Build history of the part. All positions in model axes, mm. Face numbers are marked on the shaded views. A direction names the side the tool comes from. Give positions to 0.01 mm unless a question says otherwise; leave off trailing zeros. Order: outer loops, then holes, each group sorted by start corner. A loop starts at its lowest first (then second) coordinate and runs counter-clockwise, first axis right, second up. Notation, with made-up numbers: (20.5, 64.5) - (70.5, 64.5) arc R7 cw to (70.5, 68.5) - close; hole circle Ø1 at (84, -39). An arc over 180 degrees is marked (long way). Use a Markdown table: item, result.
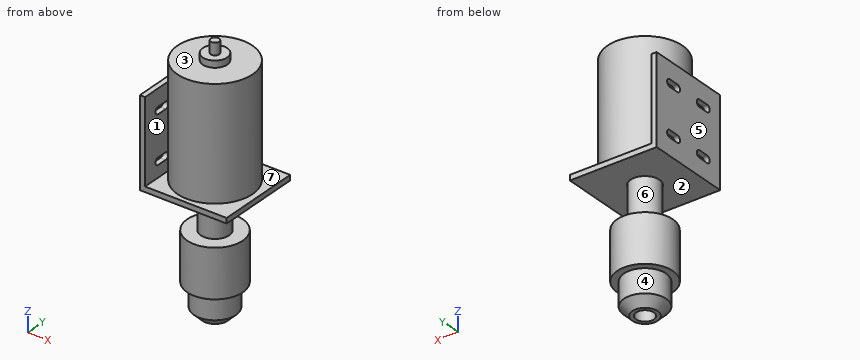
from build123d import *

# Parameters (mm, degrees)
SKETCH1_R           = 22.25
BOSS_EXTRUDE1_DEPTH = 66
SKETCH2_R           = 7.25
BOSS_EXTRUDE2_DEPTH = 4
SKETCH3_R           = 2.5
BOSS_EXTRUDE3_DEPTH = 7
SKETCH4_W           = 51.5
SKETCH4_H           = 50
SKETCH4_R           = 8.6
BOSS_EXTRUDE4_DEPTH = 3.1
SKETCH5_R           = 8.4
BOSS_EXTRUDE5_DEPTH = 27.7
SKETCH6_R           = 16.5
BOSS_EXTRUDE6_DEPTH = 28.5
SKETCH7_R           = 12.5
BOSS_EXTRUDE7_DEPTH = 18.9
SKETCH8_R           = 5.3
CUT_EXTRUDE1_DEPTH  = 26.4
CHAMFER1_SIZE       = 5
SKETCH9_W           = 3.1
SKETCH9_H           = 50
BOSS_EXTRUDE8_DEPTH = 49.3
CUT_EXTRUDE2_REACH  = 53.5


with BuildPart() as part:
    # Sketch1 → Boss-Extrude1 (new body)
    with BuildSketch(Plane.XY):
        Circle(SKETCH1_R)
    extrude(amount=BOSS_EXTRUDE1_DEPTH)

    # Sketch2 → Boss-Extrude2 (add)
    with BuildSketch(Plane.XY.offset(66)):
        Circle(SKETCH2_R)
    extrude(amount=BOSS_EXTRUDE2_DEPTH)

    # Sketch3 → Boss-Extrude3 (add)
    with BuildSketch(Plane.XY.offset(70)):
        Circle(SKETCH3_R)
    extrude(amount=BOSS_EXTRUDE3_DEPTH)

    # Sketch4 → Boss-Extrude4 (add)
    with BuildSketch(Plane(origin=(0, 0, 0), x_dir=(-1, 0, 0), z_dir=(0, 0, -1))):
        Rectangle(SKETCH4_W, SKETCH4_H)
        Circle(SKETCH4_R, mode=Mode.SUBTRACT)
    extrude(amount=BOSS_EXTRUDE4_DEPTH)

    # Sketch5 → Boss-Extrude5 (add)
    with BuildSketch(Plane(origin=(0, 0, 0), x_dir=(-1, 0, 0), z_dir=(0, 0, -1))):
        Circle(SKETCH5_R)
    extrude(amount=BOSS_EXTRUDE5_DEPTH)

    # Sketch6 → Boss-Extrude6 (add)
    with BuildSketch(Plane(origin=(0, 0, -27.7), x_dir=(-1, 0, 0), z_dir=(0, 0, -1))):
        Circle(SKETCH6_R)
    extrude(amount=BOSS_EXTRUDE6_DEPTH)

    # Sketch7 → Boss-Extrude7 (add)
    with BuildSketch(Plane(origin=(0, 0, -56.2), x_dir=(-1, 0, 0), z_dir=(0, 0, -1))):
        Circle(SKETCH7_R)
    extrude(amount=BOSS_EXTRUDE7_DEPTH)

    # Sketch8 → Cut-Extrude1 (cut)
    with BuildSketch(Plane(origin=(0, 0, -75.1), x_dir=(-1, 0, 0), z_dir=(0, 0, -1))):
        Circle(SKETCH8_R)
    extrude(amount=-CUT_EXTRUDE1_DEPTH, mode=Mode.SUBTRACT)

    # Chamfer1
    chamfer1_edges = [part.edges().sort_by_distance(p)[0] for p in [
        (12.5, 0, -75.1),
    ]]
    chamfer(chamfer1_edges, length=CHAMFER1_SIZE)

    # Sketch9 → Boss-Extrude8 (add)
    with BuildSketch(Plane.XY):
        with Locations((-24.2, 0)):
            Rectangle(SKETCH9_W, SKETCH9_H)
    extrude(amount=BOSS_EXTRUDE8_DEPTH)

    # Sketch10 → Cut-Extrude2 (cut, up to next)
    with BuildSketch(Plane.ZY.offset(25.75), mode=Mode.PRIVATE) as cut_extrude2_sk1:
        with BuildLine():
            Line((39.2, 14.7), (39.2, 8.7))
            ThreePointArc((39.2, 8.7), (37.1, 6.6), (35, 8.7))
            Line((35, 8.7), (35, 14.7))
            ThreePointArc((35, 14.7), (37.1, 16.8), (39.2, 14.7))
        make_face()
    cut_extrude2_tool1 = extrude(cut_extrude2_sk1.sketch, amount=-CUT_EXTRUDE2_REACH, mode=Mode.PRIVATE) & part.part
    add(cut_extrude2_tool1.solids().sort_by_distance((-25.75, 11.7, 37.1))[0], mode=Mode.SUBTRACT)
    # Sketch10 → Cut-Extrude2 (cut, up to next)
    with BuildSketch(Plane.ZY.offset(25.75), mode=Mode.PRIVATE) as cut_extrude2_sk2:
        with BuildLine():
            Line((39.2, -14.7), (39.2, -8.7))
            ThreePointArc((39.2, -8.7), (37.1, -6.6), (35, -8.7))
            Line((35, -8.7), (35, -14.7))
            ThreePointArc((35, -14.7), (37.1, -16.8), (39.2, -14.7))
        make_face()
    cut_extrude2_tool2 = extrude(cut_extrude2_sk2.sketch, amount=-CUT_EXTRUDE2_REACH, mode=Mode.PRIVATE) & part.part
    add(cut_extrude2_tool2.solids().sort_by_distance((-25.75, -11.7, 37.1))[0], mode=Mode.SUBTRACT)
    # Sketch10 → Cut-Extrude2 (cut, up to next)
    with BuildSketch(Plane.ZY.offset(25.75), mode=Mode.PRIVATE) as cut_extrude2_sk3:
        with BuildLine():
            Line((7, -14.7), (7, -8.7))
            ThreePointArc((7, -8.7), (9.1, -6.6), (11.2, -8.7))
            Line((11.2, -8.7), (11.2, -14.7))
            ThreePointArc((11.2, -14.7), (9.1, -16.8), (7, -14.7))
        make_face()
    cut_extrude2_tool3 = extrude(cut_extrude2_sk3.sketch, amount=-CUT_EXTRUDE2_REACH, mode=Mode.PRIVATE) & part.part
    add(cut_extrude2_tool3.solids().sort_by_distance((-25.75, -11.7, 9.1))[0], mode=Mode.SUBTRACT)
    # Sketch10 → Cut-Extrude2 (cut, up to next)
    with BuildSketch(Plane.ZY.offset(25.75), mode=Mode.PRIVATE) as cut_extrude2_sk4:
        with BuildLine():
            Line((7, 14.7), (7, 8.7))
            ThreePointArc((7, 8.7), (9.1, 6.6), (11.2, 8.7))
            Line((11.2, 8.7), (11.2, 14.7))
            ThreePointArc((11.2, 14.7), (9.1, 16.8), (7, 14.7))
        make_face()
    cut_extrude2_tool4 = extrude(cut_extrude2_sk4.sketch, amount=-CUT_EXTRUDE2_REACH, mode=Mode.PRIVATE) & part.part
    add(cut_extrude2_tool4.solids().sort_by_distance((-25.75, 11.7, 9.1))[0], mode=Mode.SUBTRACT)


solid = part.part
1) Slice it at A-A (z = 37.1). Write the cut outline in (x, y).
Computed:
| item | result |
|---|---|
| outline | (-25.75, -25) - (-22.65, -25) - (-22.65, -16.8) - (-25.75, -16.8) - close; (-25.75, -6.6) - (-22.65, -6.6) - (-22.65, 6.6) - (-25.75, 6.6) - close; (-25.75, 16.8) - (-22.65, 16.8) - (-22.65, 25) - (-25.75, 25) - close; circle Ø44.5 at (0, 0) |
2) Wall check: line 1 (Y direction, x = 0, z = -1); line 2 (Z direction, x = -15, y = 4.5); line 3 (Y direction, x = 0, z = -57.25). Give the ranges that are in metal, low to high. Write a range as from..to.
Computed:
| item | result |
|---|---|
| line 1 | y = -25..-8.6, -8.4..8.4, 8.6..25 |
| line 2 | z = -56.2..-27.7, -3.1..66 |
| line 3 | y = -12.5..-5.3, 5.3..12.5 |
3) Pin check, flat tips, straight feed: P1, Ø0.9, axis at x = -25, y = -11.5, coming from the -Z side; P2, Ø5, axis at x = -0.5, y = -3.5, coming from the -Z side; P3, Ø2.5, axis at x = -24, y = 10.5, coming from the +Z side; P4, Ø1.5, axis at x = -6, y = 11, coming from the +Z side. Stop position of each tip, or through.
Computed:
| item | result |
|---|---|
| P1 | stops at z = -3.1 |
| P2 | stops at z = -75.1 |
| P3 | stops at z = 49.3 |
| P4 | stops at z = 66 |
4) Slice it at D-D (z = -62). Write the cut outline in (x, y), and give its area (3 significant figures).
Computed:
| item | result |
|---|---|
| outline | circle Ø25 at (0, 0); hole circle Ø10.6 at (0, 0) |
| area | 403 mm² |
5) Tool access for the marked faces 1, 2, 3 and 4: list every direction of +Z, -Z, +X, -X, +Y, -Y with a clear straight run to the whole face (end or side of a thin tool).
Computed:
| item | result |
|---|---|
| face 1 | +Z, +Y, -Y |
| face 2 | none |
| face 3 | +Z |
| face 4 | -Z |
6) Slice it at B-B (z = 16). Write the cut outline in (x, y), and give its area (3 significant figures).
Computed:
| item | result |
|---|---|
| outline | (-25.75, -25) - (-22.65, -25) - (-22.65, 25) - (-25.75, 25) - close; circle Ø44.5 at (0, 0) |
| area | 1,710 mm² |
7) Two-plate mould, pull along Z, no slides. Class the marked faces 5, 6 and 7: +Z half, -Z half, draft (parallel to the pull), parting line (faces both ways), or undercut.
Computed:
| item | result |
|---|---|
| face 5 | draft |
| face 6 | undercut |
| face 7 | +Z half |
8) Slice it at C-C (x = 14). Write the cut outline in (y, z), and give its area (3 significant figures).
Computed:
| item | result |
|---|---|
| outline | (-25, -3.1) - (25, -3.1) - (25, 0) - (17.29, 0) - (17.29, 66) - (-17.29, 66) - (-17.29, 0) - (-25, 0) - close; (-8.73, -56.2) - (8.73, -56.2) - (8.73, -27.7) - (-8.73, -27.7) - close |
| area | 2,940 mm² |
